Work out the finished part from the listing and answer in its coordinate system (mm). A direction names the side the tool comes from. Give positions to 0.01 mm unless a question says otherwise; leave off trailing zeros. Loops run counter-clockwise (first coordinate to the right, second up) from the corner with the lowest first, then second, coordinate; pieces in that order, holes last. Notation, with made-up numbers: (-32.5, -12.75) - (23.5, -12.75) arc R16 ccw to (23.5, -7.75) - close; hole circle Ø5 at (-3.5, 2). An arc over 180 degrees is marked (long way). One line per item, written item: value.
from build123d import *

# Parameters (mm, degrees)
ESQUISSE1_W                     = 130
ESQUISSE1_H                     = 100
BOSS_EXTRU_1_DEPTH              = 5
ENL_V_MAT_EXTRU_3_DEPTH         = 3
R_P_TITION_LIN_AIRE1_COUNT      = 2
R_P_TITION_LIN_AIRE1_PITCH      = 58
R_P_TITION_LIN_AIRE1_COUNT_DIR2 = 2
R_P_TITION_LIN_AIRE1_PITCH_DIR2 = 49
ESQUISSE8_R                     = 2.598076211
ENL_V_MAT_EXTRU_4_DEPTH         = 93.709474566
R_P_TITION_LIN_AIRE2_COUNT      = 2
R_P_TITION_LIN_AIRE2_PITCH      = 58
R_P_TITION_LIN_AIRE2_COUNT_DIR2 = 2
R_P_TITION_LIN_AIRE2_PITCH_DIR2 = 49
ESQUISSE9_W                     = 12
ESQUISSE9_H                     = 20
BOSS_EXTRU_2_DEPTH              = 15
BOSS_EXTRU_3_DEPTH              = 20
ESQUISSE14_W                    = 16
ESQUISSE14_H                    = 7
ENL_V_MAT_EXTRU_6_DEPTH         = 16
ENL_V_MAT_EXTRU_7_DEPTH         = 13
ESQUISSE18_R                    = 1.75
ENL_V_MAT_EXTRU_8_DEPTH         = 33
CONG_1_R                        = 5
CONG_2_R                        = 5
ESQUISSE19_W                    = 21
ESQUISSE19_H                    = 14.5
ENL_V_MAT_EXTRU_9_DEPTH         = 3
ESQUISSE20_R                    = 7.25
ENL_V_MAT_EXTRU_10_DEPTH        = 12


with BuildPart() as part:
    # Esquisse1 → Boss.-Extru.1 (new body)
    with BuildSketch(Plane(origin=(0, 0, 0), x_dir=(1, 0, 0), z_dir=(0, 1, 0))):
        with Locations((12.518489284, 0.605636973)):
            Rectangle(ESQUISSE1_W, ESQUISSE1_H)
    extrude(amount=BOSS_EXTRU_1_DEPTH)

    # Esquisse5 → Enlèv. mat.-Extru.3 (cut)
    with BuildSketch(Plane(origin=(0, 5, 0), x_dir=(1, 0, 0), z_dir=(0, 1, 0))):
        Polygon((-28.974508208, 22.511616263), (-27.48152163, 25.113729073), (-28.988524137, 27.707749783), (-31.988513224, 27.699657683), (-33.481499802, 25.097544873), (-31.974497295, 22.503524163), align=None)
    enl_v_mat_extru_3 = extrude(amount=-ENL_V_MAT_EXTRU_3_DEPTH, mode=Mode.SUBTRACT)

    # Répétition linéaire1: Enl_v. mat.-Extru.3 2 × 2
    with Locations(*[(i * R_P_TITION_LIN_AIRE1_PITCH, 0, j * R_P_TITION_LIN_AIRE1_PITCH_DIR2) for i in range(R_P_TITION_LIN_AIRE1_COUNT) for j in range(R_P_TITION_LIN_AIRE1_COUNT_DIR2) if (i, j) != (0, 0)]):
        add(enl_v_mat_extru_3, mode=Mode.SUBTRACT)

    # Esquisse8 → Enlèv. mat.-Extru.4 (cut, through all)
    with BuildSketch(Plane(origin=(0, 5, 0), x_dir=(1, 0, 0), z_dir=(0, 1, 0))):
        with Locations(Location((-30.481510716, 25.105636973, 0), (0, 0, 270))):
            Circle(ESQUISSE8_R)
    enl_v_mat_extru_4 = extrude(amount=-ENL_V_MAT_EXTRU_4_DEPTH, mode=Mode.SUBTRACT)

    # Répétition linéaire2: Enl_v. mat.-Extru.4 2 × 2
    with Locations(*[(i * R_P_TITION_LIN_AIRE2_PITCH, 0, j * R_P_TITION_LIN_AIRE2_PITCH_DIR2) for i in range(R_P_TITION_LIN_AIRE2_COUNT) for j in range(R_P_TITION_LIN_AIRE2_COUNT_DIR2) if (i, j) != (0, 0)]):
        add(enl_v_mat_extru_4, mode=Mode.SUBTRACT)

    # Esquisse9 → Boss.-Extru.2 (add)
    with BuildSketch(Plane(origin=(0, 5, 0), x_dir=(1, 0, 0), z_dir=(0, 1, 0))):
        with Locations((56.884872881, 0.605636973)):
            Rectangle(ESQUISSE9_W, ESQUISSE9_H)
    extrude(amount=BOSS_EXTRU_2_DEPTH)

    # Esquisse10 → Boss.-Extru.3 (add)
    with BuildSketch(Plane.XY.offset(9.394363027)):
        with BuildLine():
            Line((50.884872881, 20), (62.884872881, 20))
            ThreePointArc((62.884872881, 20), (56.884872881, 30.605551275), (50.884872881, 20))
        make_face()
    extrude(amount=-BOSS_EXTRU_3_DEPTH)

    # Esquisse14 → Enlèv. mat.-Extru.6 (cut)
    with BuildSketch(Plane(origin=(0, 30.605551275, 0), x_dir=(1, 0, 0), z_dir=(0, 1, 0))):
        with Locations((57.018489284, 0.605636973)):
            Rectangle(ESQUISSE14_W, ESQUISSE14_H)
    extrude(amount=-ENL_V_MAT_EXTRU_6_DEPTH, mode=Mode.SUBTRACT)

    # Esquisse17 → Enlèv. mat.-Extru.7 (cut)
    with BuildSketch(Plane.XY.offset(19.394363027)):
        Polygon((60.23131756, 22.03882177), (59.914922773, 25.720292627), (56.568478094, 27.287022133), (53.538428202, 25.172280781), (53.854822989, 21.490809924), (57.201267668, 19.924080418), align=None)
    extrude(amount=-ENL_V_MAT_EXTRU_7_DEPTH, mode=Mode.SUBTRACT)

    # Esquisse18 → Enlèv. mat.-Extru.8 (cut)
    with BuildSketch(Plane.XY.offset(19.394363027)):
        with Locations((56.884872881, 23.605551275)):
            Circle(ESQUISSE18_R)
    extrude(amount=-ENL_V_MAT_EXTRU_8_DEPTH, mode=Mode.SUBTRACT)

    # Congé1
    cong_1_edges = [part.edges().sort_by_distance(p)[0] for p in [
        (50.884872881, 5, -0.605636973),
        (56.884872881, 5, 9.394363027),
        (62.884872881, 5, -0.605636973),
        (56.884872881, 5, -10.605636973),
    ]]
    fillet(cong_1_edges, radius=CONG_1_R)

    # Congé2
    cong_2_edges = [part.edges().sort_by_distance(p)[0] for p in [
        (-52.481510716, 2.5, -50.605636973),
        (77.518489284, 2.5, -50.605636973),
        (77.518489284, 2.5, 49.394363027),
        (-52.481510716, 2.5, 49.394363027),
    ]]
    fillet(cong_2_edges, radius=CONG_2_R)

    # Esquisse19 → Enlèv. mat.-Extru.9 (cut)
    with BuildSketch(Plane(origin=(0, 5, 0), x_dir=(1, 0, 0), z_dir=(0, 1, 0))):
        with Locations((3.018489284, 0.605636973)):
            Rectangle(ESQUISSE19_W, ESQUISSE19_H)
    extrude(amount=-ENL_V_MAT_EXTRU_9_DEPTH, mode=Mode.SUBTRACT)

    # Esquisse20 → Enlèv. mat.-Extru.10 (cut)
    with BuildSketch(Plane(origin=(0, 5, 0), x_dir=(1, 0, 0), z_dir=(0, 1, 0))):
        with Locations(Location((3.018489284, 0.605636973, 0), (0, 0, 270))):
            Circle(ESQUISSE20_R)
    extrude(amount=-ENL_V_MAT_EXTRU_10_DEPTH, mode=Mode.SUBTRACT)


solid = part.part
1. For faces 4 (the flat face through (11, 2, -1)), 5 (the flat face through (12, 2, -50.606)), 6 (the flat face through (57, 18, 9.394)), determine the directions among +Z, -Z, +X, -X, +Y, -Y from which every point of the face is accessible in a straight line to the end or side of a thin tool.
Output:
face 4: +Y
face 5: -Z, +X, -X, +Y, -Y
face 6: +Z, +X, -X, +Y
2. The mould has two halves that part along X. Classify faces 1 (the flat face through (12, 0, -1)), 2 (the flat face through (-28.224, 3.521, -26.393)), 3 (the cylindrical face through (57.092, 30.602, -7.31)): released by +X, released by -X, zero draft, split by the parting line, or undercut.
Output:
face 1: zero draft
face 2: undercut
face 3: split by the parting line
3. Section B-B (x = -2) is taken. Write down the section's boundary in (y, z), and give its area (3 significant figures).
Output:
outline: (0, -50.61) - (5, -50.61) - (5, -7.86) - (2, -7.86) - (2, -5.84) - (0, -5.84) - close; (0, 4.63) - (2, 4.63) - (2, 6.64) - (5, 6.64) - (5, 49.39) - (0, 49.39) - close
area: 436 mm²
4. Section D-D (x = 41.5) is taken. Write down the section's boundary in (y, z).
Output:
outline: (0, -50.61) - (5, -50.61) - (5, 49.39) - (0, 49.39) - close
5. Section C-C (z = 1) is taken. Write down the section's boundary in (x, y).
Output:
outline: (-52.48, 0) - (-4.05, 0) - (-4.05, 2) - (-7.48, 2) - (-7.48, 5) - (-52.48, 5) - close; (10.09, 0) - (77.52, 0) - (77.52, 5) - (67.88, 5) arc R5 cw to (62.88, 10) - (62.88, 14.61) - (50.88, 14.61) - (50.88, 10) arc R5 cw to (45.88, 5) - (13.52, 5) - (13.52, 2) - (10.09, 2) - close
6. Section A-A (y = 18) is taken. Write down the section's boundary in (x, z), and give its area (3 significant figures).
Output:
outline: (50.88, -10.61) - (62.88, -10.61) - (62.88, -4.11) - (50.88, -4.11) - close; (50.88, 2.89) - (62.88, 2.89) - (62.88, 9.39) - (50.88, 9.39) - close
area: 156 mm²
7. Flat-ended cylindrical pins translate along their axes: pin 1 Ø1 at (x, y) = (57.5, 6) entering from -Z; pin 2 Ø0.6 at (x, z) = (25, -25) entering from +Y; pin 3 Ø3 at (y, z) = (13.5, 0.5) entering from -X; pin 4 Ø1 at (x, z) = (-17, -6) entering from -Y. Find the tip coordinate at first contact, or state that the pin passes through.
Output:
pin 1: stops at z = -13.43
pin 2: stops at y = 2
pin 3: stops at x = 50.88
pin 4: stops at y = 0
8. Find the intervals of material crossed by line 1 along Z through (x, y) = (59, 18); line 2 along X through (y, z) = (14, -10.5); line 3 along Y through (x, z) = (40, -40), in increasing order.
Output:
line 1: z = -10.61 to -4.11, 2.89 to 9.39
line 2: x = 50.88 to 62.88
line 3: y = 0 to 5
